The listing builds one solid part. Answer for the finished solid, in the listing's coordinates (mm). A direction names the side the tool comes from. Coordinates: 2 decimals unless noted, no trailing zeros. Loops run counter-clockwise (first coordinate to the right, second up) from the corner with the lowest first, then second, coordinate; pieces in that order, holes last. Notation, with made-up numbers: (75.25, 20.5) - (127.25, 20.5) arc R15 ccw to (127.25, 29.5) - close; hole circle Ø5 at (18, 22.5). An arc over 180 degrees is marked (long way). Use one line per item in the form item = value. Start each with the question number.
```python
from build123d import *

# Parameters (mm, degrees)
SKETCH2_R          = 4
CUT_EXTRUDE1_DEPTH = 10
SKETCH3_R          = 4
CUT_EXTRUDE2_DEPTH = 18


with BuildPart() as part:
    # Sketch1 → Revolve1 (revolve)
    with BuildSketch(Plane.XY, mode=Mode.PRIVATE) as revolve1_sk:
        Polygon((-15, 17.7), (-15, 37.7), (-14.2, 37.7), (-14.2, 18.5), (0, 18.5), (0, 17.7), align=None)
    revolve(revolve1_sk.sketch.rotate(Axis((0, 0, 0), (0, 1, 0)), 270), axis=Axis((0, 0, 0), (0, 1, 0)))

    # Sketch2 → Cut-Extrude1 (cut)
    with BuildSketch(Plane(origin=(0, 18.5, 0), x_dir=(1, 0, 0), z_dir=(0, 1, 0))):
        with Locations(Location((0, 0, 0), (0, 0, 270))):
            Circle(SKETCH2_R)
    extrude(amount=-CUT_EXTRUDE1_DEPTH, mode=Mode.SUBTRACT)

    # Sketch3 → Cut-Extrude2 (cut)
    with BuildSketch(Plane(origin=(0, 0, 0), x_dir=(0, 0, -1), z_dir=(1, 0, 0))):
        with Locations((0, 27.7)):
            Circle(SKETCH3_R)
    extrude(amount=-CUT_EXTRUDE2_DEPTH, mode=Mode.SUBTRACT)


solid = part.part
```
(1) For faces 1 (the face through (5.5, 37.7, -13.3)), 2 (the face through (3, 18.5, -3)), determine the directions among +Z, -Z, +X, -X, +Y, -Y from which every point of the face is accessible in a straight line to the end or side of a thin tool.
(2) Determine the mould class of faces 3 (the face through (14.643, 27.84, 3.252)), 4 (the face through (-14.3, 25.3, 3.2)), 5 (the face through (3, 17.7, 3)) for opening direction Z: +Z half, -Z half, draft (parallel to the pull), parting line (faces both ways), or undercut.
(3) A cutting plane is placed at A-A (x = 0). Determine the outline of the cut face in (y, z).
(4) A cutting plane is placed at C-C (x = 10.5). Determine the outline of the cut face in (y, z).
(5) A cutting plane is placed at D-D (z = -9.5). Determine the outline of the cut face in (x, y).
(6) Each of these flat-tipped pins is pushed along its axis until it touches: pin 1 Ø5 at (x, y) = (3.5, 32.5) entering from +Z; pin 2 Ø8 at (y, z) = (32, 11.5) entering from +X; pin 3 Ø1 at (y, z) = (22.5, 5.5) entering from -X; pin 4 Ø7 at (x, z) = (0, 0) entering from -Y. Where does it stop, or does it pass through?
(7) A cutting plane is placed at B-B (z = 0). Determine the outline of the cut face in (x, y), then the cut area to 3 significant figures.
(8) Find the intervals of material crossed by probe 1 along X at (y, z) = (17.9, 0); probe 2 along Y at (x, z) = (1.5, -7); probe 3 along X at (y, z) = (34.5, -6), in increasing order. Write a range as from..to.
Evaluation:
q1.face_1 = +Z, -Z, +X, -X, +Y
q1.face_2 = +Y
q2.face_3 = parting line
q2.face_4 = undercut
q2.face_5 = draft
q3.outline = (17.7, -15) - (37.7, -15) - (37.7, -14.2) - (18.5, -14.2) - (18.5, -4) - (17.7, -4) - close; (17.7, 4) - (18.5, 4) - (18.5, 14.2) - (37.7, 14.2) - (37.7, 15) - (17.7, 15) - close
q4.outline = (17.7, -10.71) - (37.7, -10.71) - (37.7, -9.56) - (18.5, -9.56) - (18.5, 9.56) - (37.7, 9.56) - (37.7, 10.71) - (17.7, 10.71) - close
q5.outline = (-11.61, 17.7) - (11.61, 17.7) - (11.61, 37.7) - (10.55, 37.7) - (10.55, 18.5) - (-10.55, 18.5) - (-10.55, 37.7) - (-11.61, 37.7) - close
q6.pin_1 = 14.97
q6.pin_2 = 12.99
q6.pin_3 = -14.14
q6.pin_4 = through
q7.outline = (-15, 17.7) - (-4, 17.7) - (-4, 18.5) - (-14.2, 18.5) - (-14.2, 23.7) - (-15, 23.7) - close; (-15, 31.7) - (-14.2, 31.7) - (-14.2, 37.7) - (-15, 37.7) - close; (4, 17.7) - (15, 17.7) - (15, 37.7) - (14.2, 37.7) - (14.2, 18.5) - (4, 18.5) - close
q7.area = 41.9 mm^2
q8.probe_1 = -15..-4, 4..15
q8.probe_2 = 17.7..18.5
q8.probe_3 = -13.75..-12.87, 12.87..13.75
